Could you check a few things on this model? Use its own coordinates, in mm. Coordinates: 2 decimals unless noted, no trailing zeros. Loops run counter-clockwise (first coordinate to the right, second up) from the corner with the lowest first, then second, coordinate; pieces in that order, holes last. Notation, with made-up numbers: M -10.5,54.5 L 44.5,54.5 A20 ccw 44.5,68.5 Z; hole C 30.5,-1 d6. An arc over 180 degrees is marked long. Write each question's results on one line, items separated by ' | '.
Autodesk Inventor part; units mm, degrees
ref_plane "YZ Plane" through (0, 0, 0) normal (1, 0, 0) x (0, 1, 0)
ref_plane "XZ Plane" through (0, 0, 0) normal (0, 1, 0) x (-1, 0, 0)
ref_plane "XY Plane" through (0, 0, 0) normal (0, 0, 1) x (1, 0, 0)
sketch "Sketch1" plane through (0, 0, 0) normal (0, 0, 1) x (1, 0, 0)
  line L0 (0, 0) -> (80, 0)
  line L1 (80, 0) -> (80, 25)
  line L2 (80, 25) -> (0, 25)
  line L3 (0, 25) -> (0, 0)
  point P0 (14.5, 12.5)
  point P1 (65.5, 12.5)
  dimension "d0" = 80
  dimension "d1" = 25
  dimension "d2" = 12.5
  dimension "d3" = 14.5
  dimension "d4" = 51
extrude "Extrusion1" add sketch "Sketch1" along normal blind 5
sketch "Sketch2" plane through (0, 0, 0) normal (0, 0, 1) x (1, 0, 0)
  line L0 (0, 0) -> (80, 0)
  line L1 (80, 0) -> (80, 25)
  line L2 (80, 25) -> (0, 25)
  line L3 (0, 25) -> (0, 0)
  point P0 (14.5, 12.5)
  point P1 (65.5, 12.5)
  dimension "d5" = 80
  dimension "d6" = 25
  dimension "d7" = 12.5
  dimension "d8" = 14.5
  dimension "d9" = 51
hole "Hole1" at (14.5, 12.5, 0) at (65.5, 12.5, 0) direction (0, 0, 1) diameter 3.5 end through all
fillet "Fillet1" radius 2 4 edges at (0, 25, 2.5) (80, 25, 2.5) (80, 0, 2.5) (0, 0, 2.5)
sketch "Sketch3" plane through (0, 0, 5) normal (0, 0, 1) x (1, 0, 0)
  arc A0 (0, 2) -> (2, 0) centre (2, 2) ccw
  line L0 (2, 0) -> (78, 0)
  arc A1 (78, 0) -> (80, 2) centre (78, 2) ccw
  line L1 (80, 2) -> (80, 23)
  arc A2 (80, 23) -> (78, 25) centre (78, 23) ccw
  line L2 (78, 25) -> (2, 25)
  arc A3 (2, 25) -> (0, 23) centre (2, 23) ccw
  line L3 (0, 23) -> (0, 2)
  circle A4 centre (14.5, 12.5) radius 1.75
  circle A5 centre (65.5, 12.5) radius 1.75
  point P0 (0, 0)
properties part number "BasePatasVTOL"
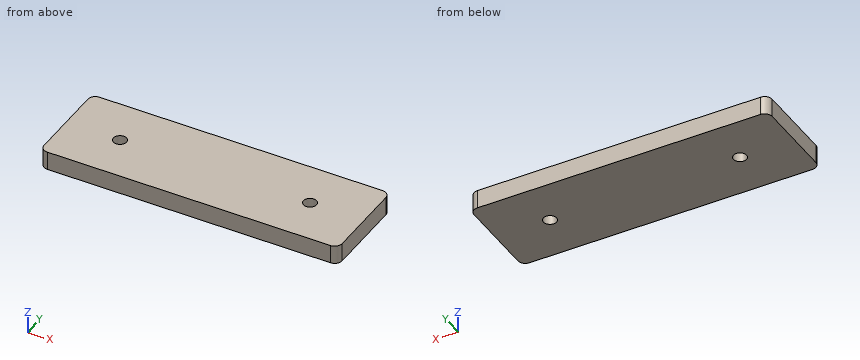
(1) Imagine slicing it at B-B, the plane y = 12.5. List the corners of the cut face in (x, z) for me, and give its area (3 significant figures).
Reported:
outline: M 0,0 L 12.75,0 L 12.75,5 L 0,5 Z; M 16.25,0 L 63.75,0 L 63.75,5 L 16.25,5 Z; M 67.25,0 L 80,0 L 80,5 L 67.25,5 Z | area: 365 mm2
(2) Imagine slicing it at A-A, the plane x = 65.5. List the corners of the cut face in (y, z) for me, and give its area (4 significant figures).
Reported:
outline: M 0,0 L 10.75,0 L 10.75,5 L 0,5 Z; M 14.25,0 L 25,0 L 25,5 L 14.25,5 Z | area: 107.5 mm2
(3) Please list where these lines run through material, in increasing order: probe 1 along X at (y, z) = (12.5, 3.25); probe 2 along Y at (x, z) = (65.5, 1.8); probe 3 along X at (y, z) = (23.75, 0.55). Write a range as from..to.
Reported:
probe 1: x = 0..12.75, 16.25..63.75, 67.25..80 | probe 2: y = 0..10.75, 14.25..25 | probe 3: x = 0.15..79.85
